Input: dimensioned drawing with shaded views. Units: mm. Origin: part minimum x, y, z. Round coordinates to 2 decimals unless told otherwise and drop trailing zeros. Order: outer loops, then holes, each group sorted by start corner. A loop starts at its lowest first (then second) coordinate and runs counter-clockwise, first axis right, second up. Notation, with made-up numbers: (85.5, 41) - (103.5, 41) arc R30 cw to (103.5, 65) - close; hole circle Ø8 at (-34, 57). An arc over 180 degrees is marked (long way). Return JSON: item names as keys, results as strings. Group by question number.
1) Ray query, line 1 (X direction, y = 3.25, z = 11) (1 decimal); line 2 (Z direction, x = 2.5, y = 2.75); line 3 (X direction, y = 2.5, z = 27.5). Return the intervals inside material, ascending. Write a range as from..to.
2) Section C-C, the plane x = 1.25. Return loops of the section in (y, z), plus the area to 3 significant figures.
3) Section B-B, the plane y = 5.5. Return loops of the section in (x, z).
4) Contact query for flat-ended pins moving along their axis: P1, Ø3.5, axis at x = 3.175, y = 3.175, coming from the +Z side; P2, Ø2.5, axis at x = 3.175, y = 3.175, coming from the +Z side. Output: stop coordinate, or through.
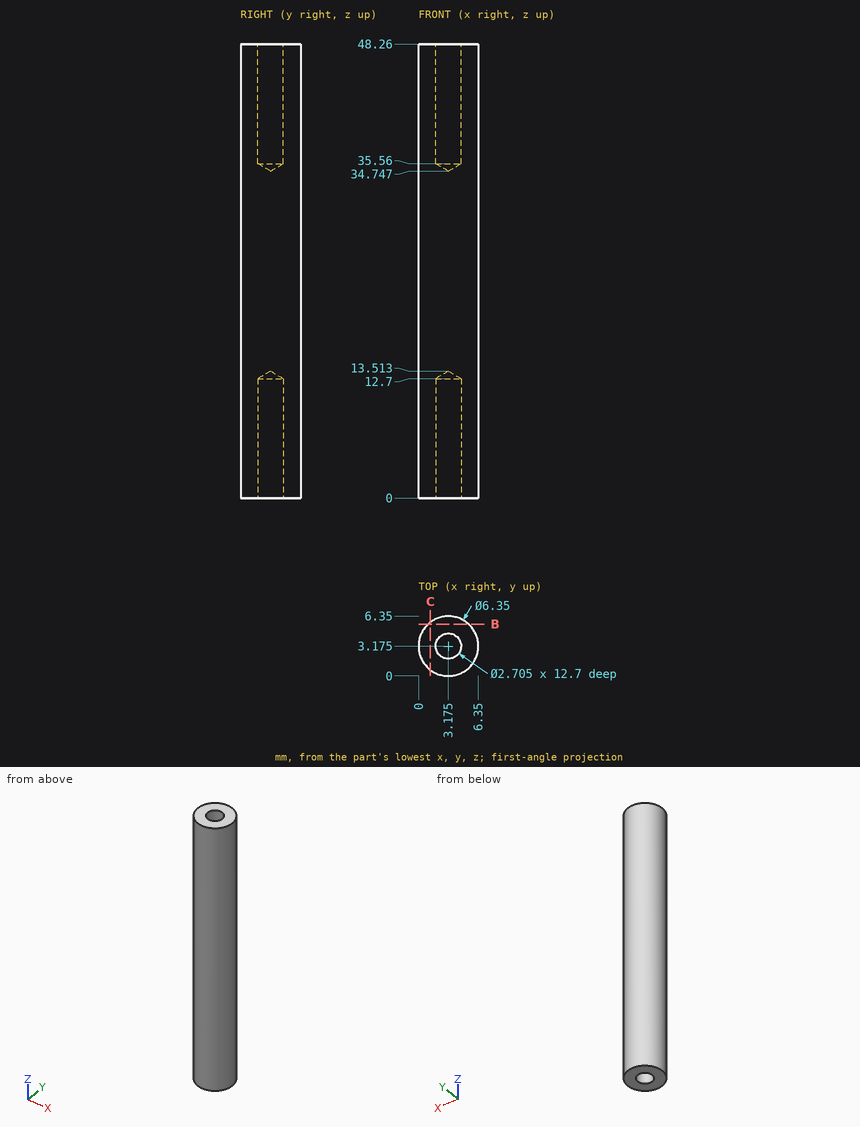
Geometry check:
{
 "1": {"line 1": "0..1.8, 4.5..6.3", "line 2": "13.03..35.23", "line 3": "0.07..6.28"},
 "2": {"outline": "(0.65, 0) - (5.7, 0) - (5.7, 48.26) - (0.65, 48.26) - close", "area": "244 mm2"},
 "3": {"outline": "(1.01, 0) - (5.34, 0) - (5.34, 48.26) - (1.01, 48.26) - close"},
 "4": {"P1": "z = 48.26", "P2": "z = 35.5"}
}
